Autodesk Inventor part; units mm, degrees
ref_plane "Work Plane1" through (-49.9795, 1.4309, 0) normal (-0.9996, 0.0286, 0) x (-0.0286, -0.9996, 0)
ref_plane "YZ Plane" through (0, 0, 0) normal (1, 0, 0) x (0, 1, 0)
ref_plane "XZ Plane" through (0, 0, 0) normal (0, 1, 0) x (-1, 0, 0)
sketch "Sketch1" plane through (0, 0, 0) normal (0, 0, 1) x (1, 0, 0)
  arc A0 (-49.9795, 1.4309) -> (49.9795, 1.4309) centre (0, 0) ccw
  line L0 (-49.9795, 1.4309) -> (-40, 350)
  line L1 (-40, 350) -> (40, 350)
  line L2 (40, 350) -> (49.9795, 1.4309)
  point P0 (0, 350)
  dimension "d0" = 100
  dimension "d1" = 350
  dimension "d2" = 80
extrude "Extrusion1" add sketch "Sketch1" along normal blind 40
sketch "Sketch2" plane through (0, 0, 0) normal (0, 0, -1) x (-1, 0, 0)
  circle A0 centre (0, 0) radius 40
  dimension "d5" = 80
extrude "Extrusion2" cut sketch "Sketch2" against normal blind 20
sketch "Sketch3" plane through (0, 0, 20) normal (0, 0, -1) x (-1, 0, 0)
  circle A0 centre (0, 0) radius 2.5
  dimension "d8" = 5
extrude "Extrusion3" cut sketch "Sketch3" against normal blind 20
sketch "Sketch4" plane through (40, 350, 40) normal (0.9996, 0.0286, 0) x (0, 0, -1)
  point P0 (40, -348.7119)
ref_plane "Work Plane1" through (-49.9795, 1.4309, 0) normal (-0.9996, 0.0286, 0) x (-0.0286, -0.9996, 0)
sketch "Sketch5" plane through (-49.9795, 1.4309, 0) normal (-0.9996, 0.0286, 0) x (-0.0286, -0.9996, 0)
  point P0 (0, 0)
sketch "Sketch6" plane through (-49.9795, 1.4309, 0) normal (-0.9996, 0.0286, 0) x (-0.0286, -0.9996, 0)
  line L0 (0, -8) -> (0, 48)
  line L1 (-348.7119, 40) -> (0, 40)
  line L2 (-348.7119, 0) -> (0, 0)
  line L3 (-188.7119, 30) -> (-328.7119, 30)
  line L4 (-328.7119, 30) -> (-328.7119, 10)
  line L5 (-328.7119, 10) -> (-188.7119, 10)
  line L6 (-188.7119, 10) -> (-188.7119, 30)
  line L7 (-348.7119, 0) -> (-348.7119, 40)
  point P0 (-348.7119, 20)
  point P1 (-328.7119, 20)
  dimension "d12" = 20
  dimension "d13" = 20
  dimension "d14" = 140
  dimension "d15" = 20
extrude "Extrusion4" cut sketch "Sketch6" against normal through all contours L6 L5 L4 L3
sketch "Sketch7" plane through (-40, 350, 0) normal (0, 1, 0) x (1, 0, 0)
  line L0 (0, -20) -> (80, -20)
  circle A0 centre (40, -20) radius 2.5
  point P0 (40, 0)
  dimension "d18" = 5
extrude "Extrusion5" cut sketch "Sketch7" against normal blind 30
fillet "Fillet1" radius 6.858 3 edges at (0, -50, 40) (44.9898, 175.7155, 40) (-44.9898, 175.7155, 40)
properties part number "Robot_arm_2"
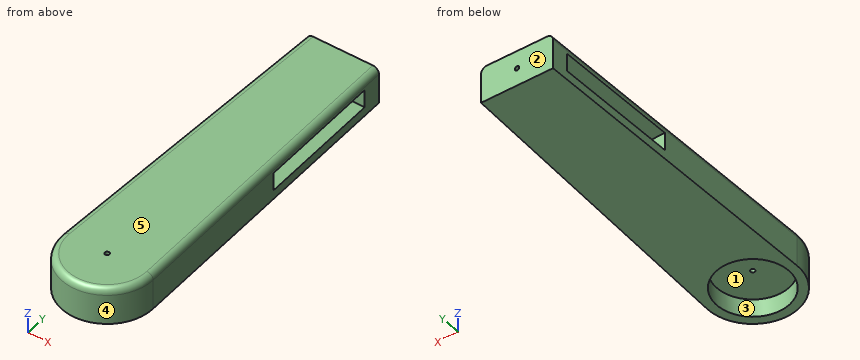
Verification items for the finished model (mm, model axes). Face numbers are marked on the shaded views. A direction names the side the tool comes from. Round coordinates to 2 decimals unless told otherwise and drop trailing zeros. Loops run counter-clockwise (first coordinate to the right, second up) from the corner with the lowest first, then second, coordinate; pieces in that order, holes last. Notation, with made-up numbers: (73.25, -35) -> (101.25, -35) arc R18 ccw to (101.25, -13) -> close; hole circle Ø9 at (-25.5, 6.25). An arc over 180 degrees is marked (long way). Answer as a JSON object with one key per item and string values.
Q1. Section check A-A (z = 36.5). Record the boundary of the cut face in (x, y).
Data:
{"outline": "(-49.1, 1.41) arc R49.12 ccw (long way) to (49.1, 1.41) -> (39.12, 350) -> (-39.12, 350) -> close; hole circle Ø5 at (0, 0)"}
Q2. Go/stop test with flat-tipped pins: P1, Ø6, axis at y = 294.5, z = 6, coming from the -X side; P2, Ø8, axis at x = 0, y = 0, coming from the -Z side; P3, Ø6.5, axis at x = 0, z = 20, coming from the -Y side. Record where each tip stops, or that it passes through.
Data:
{"P1": "stops at x = -41.67", "P2": "stops at z = 20", "P3": "stops at y = -50"}
Q3. Scan lines: line 1 (Y direction, x = 0, z = 31); line 2 (Y direction, x = 0, z = 14.75); line 3 (Z direction, x = 0, y = 345). Record each from-to range of solid material in increasing order. Write a range as from..to.
Data:
{"line 1": "y = -50..-2.5, 2.5..350", "line 2": "y = -50..-40, 40..188.79, 328.85..350", "line 3": "z = 0..17.5, 22.5..40"}
Q4. Access from +Z, -Z, +X, -X, +Y, -Y to the whole of each face (thin tool, end or side, straight path). Record for the marked faces 1 and 2.
Data:
{"face 1": "-Z", "face 2": "+Z, -Z, +X, -X, +Y"}
Q5. Draft check along X on the marked faces 3, 4 and 5. Enter one of: pulls with the +X half, pulls with the -X half, needs draft (parallel to the pull), parting line crosses it, or undercut.
Data:
{"face 3": "undercut", "face 4": "parting line crosses it", "face 5": "needs draft"}
